```python
from build123d import *

# Parameters (mm, degrees)
F1_DEPTH = 57
F0_W     = 54
F0_H     = 14
F2_DEPTH = 2
F3_START = 51
F3_DEPTH = 6
F4_W     = 40
F4_H     = 4
F5_DEPTH = 5
F6_R     = 4.99999
F7_W     = 52
F7_H     = 1
F8_DEPTH = 2
F9_START = -56
F9_DEPTH = 2


# Not quite as in the source:
# - a fillet or chamfer is up to 0.001 mm smaller than in the source, because OpenCascade refuses the exact size


with BuildPart() as f1:
    # F0 (on Front) → F1 (new body)
    with BuildSketch(Plane.XZ):
        Polygon((-59.5397581918, 21.3998371276), (-61.5397581918, 21.3998371276), (-61.5397581918, 5.3998371276), (-3.5397581918, 5.3998371276), (-3.5397581918, 21.3998371276), (-5.5397581918, 21.3998371276), (-5.5397581918, 7.3998371276), (-59.5397581918, 7.3998371276), align=None)
    extrude(amount=F1_DEPTH)

    # F0 (on Front) → F2 (join)
    with BuildSketch(Plane.XZ):
        with Locations((-32.5397581918, 14.3998371276)):
            Rectangle(F0_W, F0_H)
    extrude(amount=F2_DEPTH)

    # F0 (on Front) → F3 (join)
    with BuildSketch(Plane.XZ.offset(F3_START)):
        with Locations((-32.5397581918, 14.3998371276)):
            Rectangle(F0_W, F0_H)
    extrude(amount=F3_DEPTH)

    # F4 (on face) → F5 (cut)
    with BuildSketch(Plane.XZ.offset(57)):
        with Locations((-32.5397581918, 17.3998371276)):
            Rectangle(F4_W, F4_H)
        with Locations((-32.5397581918, 9.3998371276)):
            Rectangle(F4_W, F4_H)
    extrude(amount=-F5_DEPTH, mode=Mode.SUBTRACT)

    # F6 (radius 5 in the source; OpenCascade refuses exactly that, so slightly less here)
    f6_edges = [f1.edges().sort_by_distance(p)[0] for p in [
        (-52.539758, -52, 17.399837),
        (-52.539758, -52, 9.399837),
        (-12.539758, -52, 17.399837),
        (-12.539758, -52, 9.399837),
    ]]
    fillet(f6_edges, radius=F6_R)

    # F7 (on face) → F8 (cut)
    with BuildSketch(Plane(origin=(-61.5397581918, 0, 0), x_dir=(0, -1, 0), z_dir=(-1, 0, 0))):
        with Locations((26, 5.8998371276)):
            Rectangle(F7_W, F7_H)
    extrude(amount=-F8_DEPTH, mode=Mode.SUBTRACT)

    # F7 (on face) → F9 (cut)
    with BuildSketch(Plane(origin=(-61.5397581918, 0, 0), x_dir=(0, -1, 0), z_dir=(-1, 0, 0)).offset(F9_START)):
        with Locations((26, 5.8998371276)):
            Rectangle(F7_W, F7_H)
    extrude(amount=-F9_DEPTH, mode=Mode.SUBTRACT)


solid = f1.part
```
Part model, mm, in its own coordinate system. A direction names the side the tool comes from. Round coordinates to 2 decimals unless told otherwise and drop trailing zeros. Order: outer loops, then holes, each group sorted by start corner. A loop starts at its lowest first (then second) coordinate and runs counter-clockwise, first axis right, second up. Notation, with made-up numbers: M 45.25,-36.75 L 80.25,-36.75 A13 cw 80.25,-18.75 Z; hole C 29.5,-20 d4. An arc over 180 degrees is marked long. Put each result on its own line as item: value. Start each with the question number.
1. Drop flat-ended pins along their axis: pin 1 (0.6 mm diameter, centred on x = -5, y = -34, fed in from -Z); pin 2 (3 mm diameter, centred on x = -29, z = 17, fed in from -Y); pin 3 (1 mm diameter, centred on x = -45.5, y = -32.5, fed in from +Z). Give the stop position or say it passes through.
2. Slice it at B-B on x = -34. List the corners of the cut face in (y, z), then the cut area to 3 significant figures.
3. Drill centre lines: probe 1 along Y at (x, z) = (-23, 12.5); probe 2 along Y at (x, z) = (-41.5, 9.5); probe 3 along X at (y, z) = (-16, 8). Where is each one in solid material? Low to high. Write a range as [from, to].
4. Two-plate mould, pull along Z, no slides. Class faces 1 (the face through (-61, -26, 6.4)), 2 (the face through (-33, -2, 14)), 3 (the face through (-51.11, -53.5, 9.43)): +Z half, -Z half, draft (parallel to the pull), parting line (faces both ways), or undercut.
5. Slice it at C-C on y = -33. List the corners of the cut face in (x, z), then the cut area to 3 significant figures.
6. Slice it at D-D on z = 13.5. List the corners of the cut face in (x, y), then the cut area to 3 significant figures.
7. Tool access for faces 4 (the face through (-33, -55, 11.4)), 5 (the face through (-33, -52, 21.4)), 6 (the face through (-59.54, -26, 14)): list every direction of +Z, -Z, +X, -X, +Y, -Y with a clear straight run to the whole face (end or side of a thin tool).
Findings:
1. pin 1: z = 6.4
1. pin 2: y = -52
1. pin 3: z = 7.4
2. outline: M -57,5.4 L 0,5.4 L 0,21.4 L -2,21.4 L -2,7.4 L -51,7.4 L -51,21.4 L -57,21.4 L -57,19.4 L -52,19.4 L -52,15.4 L -57,15.4 L -57,11.4 L -52,11.4 L -52,7.4 L -57,7.4 Z
2. area: 186 mm2
3. probe 1: [-57, -51], [-2, 0]
3. probe 2: [-52, -51], [-2, 0]
3. probe 3: [-61.54, -59.54], [-5.54, -3.54]
4. face 1: -Z half
4. face 2: draft
4. face 3: undercut
5. outline: M -61.54,6.4 L -59.54,6.4 L -59.54,5.4 L -5.54,5.4 L -5.54,6.4 L -3.54,6.4 L -3.54,21.4 L -5.54,21.4 L -5.54,7.4 L -59.54,7.4 L -59.54,21.4 L -61.54,21.4 Z
5. area: 168 mm2
6. outline: M -61.54,-57 L -3.54,-57 L -3.54,0 L -61.54,0 Z; hole M -59.54,-51 L -5.54,-51 L -5.54,-2 L -59.54,-2 Z
6. area: 660 mm2
7. face 4: -Y
7. face 5: +Z, +X, -X, +Y, -Y
7. face 6: +Z
